Source: three-view drawing plus pictorial views. Frame: mm from the lowest corner of the part. Give positions to 0.01 mm unless a question says otherwise; leave off trailing zeros. Write each loop counter-clockwise with the first axis right and the second up, starting at its lowest first coordinate (ties: lowest second). Pieces come first, ordered by that corner, then holes.
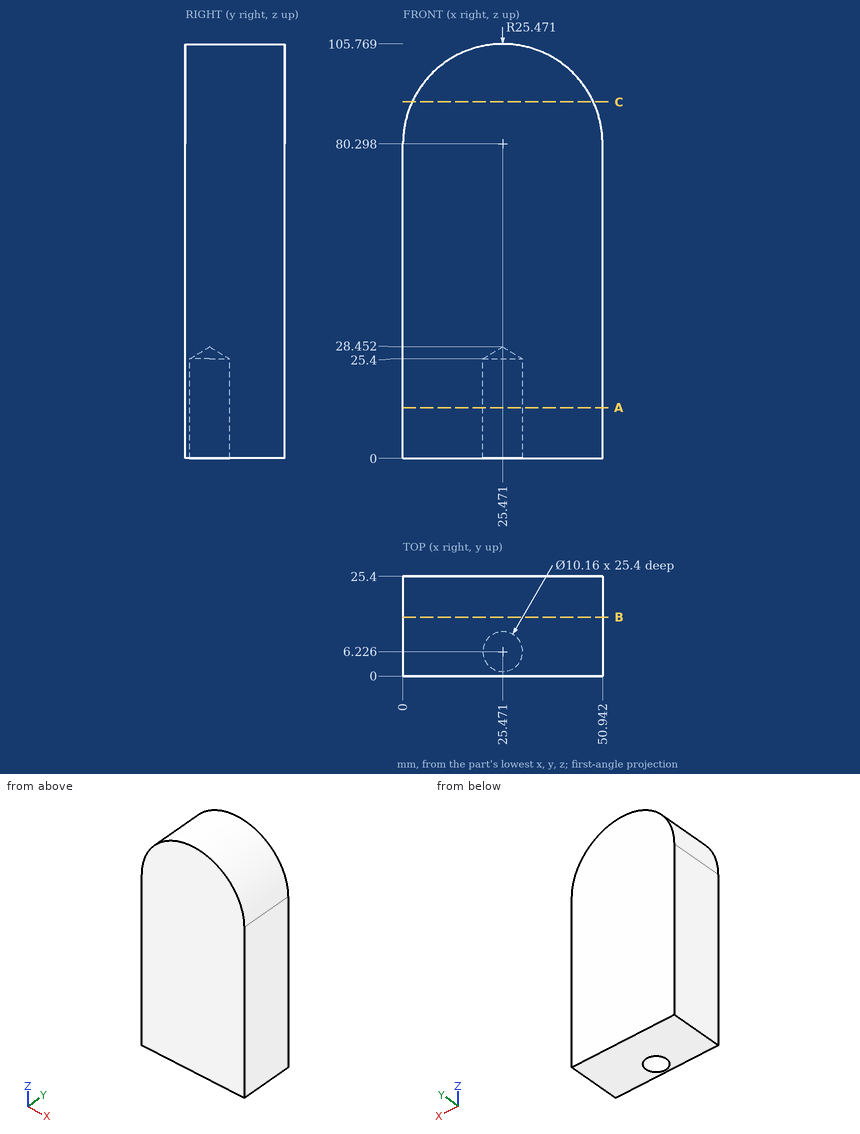
Q1. Section B-B on y = 15. Output: boundary loops of the cut face in (x, z).
Filled sheet:
outline: (0, 0) - (50.94, 0) - (50.94, 80.3) arc R25.47 ccw to (0, 80.3) - close
Q2. Ray query, line 1 along X through (y, z) = (3.75, 9) (1 decimal); line 2 along X through (y, z) = (8.5, 21) (1 decimal); line 3 along Z through (x, y) = (33, 10.5). Return the intervals inside material, ascending.
Filled sheet:
line 1: x = 0 to 21, 29.9 to 50.9
line 2: x = 0 to 20.9, 30 to 50.9
line 3: z = 0 to 104.63
Q3. Section C-C on z = 91. Output: boundary loops of the cut face in (x, y), plus the area to 3 significant figures.
Filled sheet:
outline: (2.36, 0) - (48.58, 0) - (48.58, 25.4) - (2.36, 25.4) - close
area: 1,170 mm2
Q4. Pin query (flat end, axial travel): P1, Ø8, axis at x = 25.47, y = 6.23, coming from the -Z side; P2, Ø4, axis at x = 9.5, y = 5.5, coming from the +Z side (1 decimal); P3, Ø4, axis at x = 45, y = 15.5, coming from the +Z side. Return the tip coordinate at first contact, or that it passes through.
Filled sheet:
P1: stops at z = 26.05
P2: stops at z = 101.6
P3: stops at z = 98.78
Q5. Section A-A on z = 13. Output: boundary loops of the cut face in (x, y), plus the area to 3 significant figures.
Filled sheet:
outline: (0, 0) - (50.94, 0) - (50.94, 25.4) - (0, 25.4) - close; hole circle Ø10.16 at (25.47, 6.23)
area: 1,210 mm2
